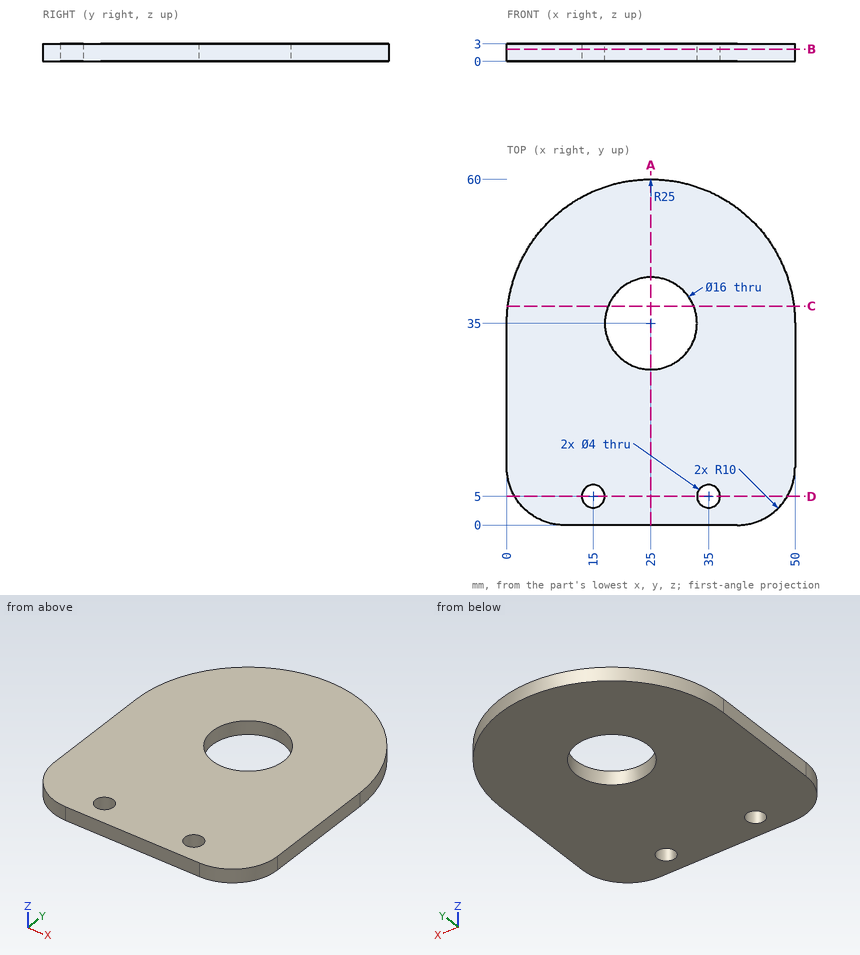
Design review of the part shown in the three views and the two pictorial views. Dimensions are in mm from the part's minimum x, y and z. Coordinates: 2 decimals unless noted, no trailing zeros. Loops run counter-clockwise (first coordinate to the right, second up) from the corner with the lowest first, then second, coordinate; pieces in that order, holes last.
(1) Consider section A-A, the plane x = 25. Give the boundary of the cut face in (y, z), plus the area to 3 significant figures.
Determined:
outline: (0, 0) - (27, 0) - (27, 3) - (0, 3) - close; (43, 0) - (60, 0) - (60, 3) - (43, 3) - close
area: 132 mm2
(2) Consider section B-B, the plane z = 2.1. Give the boundary of the cut face in (x, y).
Determined:
outline: (0, 10) arc R10 ccw to (10, 0) - (40, 0) arc R10 ccw to (50, 10) - (50, 35) arc R25 ccw to (0, 35) - close; hole circle Ø4 at (15, 5); hole circle Ø16 at (25, 35); hole circle Ø4 at (35, 5)
(3) Consider section C-C, the plane y = 38. Give the boundary of the cut face in (x, z).
Determined:
outline: (0.18, 0) - (17.58, 0) - (17.58, 3) - (0.18, 3) - close; (32.42, 0) - (49.82, 0) - (49.82, 3) - (32.42, 3) - close
(4) Wall thickness on L1, parallel to X at y = 28.5, z = 2.5; L2, parallel to Y at x = 30, z = 1.8 (3 decimals); L3, parallel to X at y = 39, z = 0.9: over which ranges is each line inside the solid? List them lowest first.
Determined:
L1: x = 0 to 20.34, 29.66 to 50
L2: y = 0 to 28.755, 41.245 to 59.495
L3: x = 0.32 to 18.07, 31.93 to 49.68
(5) Consider section D-D, the plane y = 5. Give the boundary of the cut face in (x, z).
Determined:
outline: (1.34, 0) - (13, 0) - (13, 3) - (1.34, 3) - close; (17, 0) - (33, 0) - (33, 3) - (17, 3) - close; (37, 0) - (48.66, 0) - (48.66, 3) - (37, 3) - close
